Can you work these out from the model? Positions are in its coordinate system, mm. A direction names the side the tool comes from. Round coordinates to 2 decimals unless told otherwise and drop trailing zeros. Loops run counter-clockwise (first coordinate to the right, second up) from the corner with the lowest first, then second, coordinate; pieces in that order, holes last. Notation, with made-up numbers: (53.5, 8.5) -> (78.5, 8.5) arc R21 cw to (78.5, 34.5) -> close; hole circle Ø2 at (10.5, -16.5). An arc over 180 degrees is marked (long way). Write item = value, one per line.
from build123d import *

# Parameters (mm, degrees)
CYLINDER1707_R     = 1.5
CYLINDER1707_DEPTH = 60
CYLINDER1708_R     = 1.5
CYLINDER1708_DEPTH = 60
CYLINDER1704_R     = 1.5
CYLINDER1704_DEPTH = 60
CYLINDER1705_R     = 1.5
CYLINDER1705_DEPTH = 60
BOX662_W           = 6
BOX662_H           = 6
BOX662_DEPTH       = 2
BOX664_W           = 6
BOX664_H           = 6
BOX664_DEPTH       = 2
BOX663_W           = 6
BOX663_H           = 6
BOX663_DEPTH       = 2
BOX661_W           = 6
BOX661_H           = 6
BOX661_DEPTH       = 2
CYLINDER1700_R     = 5
CYLINDER1700_DEPTH = 5
CYLINDER1699_R     = 3
CYLINDER1699_DEPTH = 48
BOX660_W           = 42
BOX660_H           = 20
BOX660_DEPTH       = 6


with BuildPart() as obj1:
    # Cylinder1707 → Cylinder1707 (new body)
    with BuildSketch(Plane(origin=(18, 85, -57), x_dir=(1, 0, 0), z_dir=(0, 0, 1))):
        Circle(CYLINDER1707_R)
    extrude(amount=CYLINDER1707_DEPTH)


with BuildPart() as obj2:
    # Cylinder1708 → Cylinder1708 (new body)
    with BuildSketch(Plane(origin=(-18, 85, -57), x_dir=(1, 0, 0), z_dir=(0, 0, 1))):
        Circle(CYLINDER1708_R)
    extrude(amount=CYLINDER1708_DEPTH)


with BuildPart() as obj3:
    # Cylinder1704 → Cylinder1704 (new body)
    with BuildSketch(Plane(origin=(-18, 95, -57), x_dir=(1, 0, 0), z_dir=(0, 0, 1))):
        Circle(CYLINDER1704_R)
    extrude(amount=CYLINDER1704_DEPTH)


with BuildPart() as compound849:
    # Cylinder1705 → Cylinder1705 (new body)
    with BuildSketch(Plane(origin=(18, 95, -57), x_dir=(1, 0, 0), z_dir=(0, 0, 1))):
        Circle(CYLINDER1705_R)
    extrude(amount=CYLINDER1705_DEPTH)

    # Compound849: union obj1, obj2, obj3
    add(obj1.part)
    add(obj2.part)
    add(obj3.part)


with BuildPart() as krychle662:
    # Box662 → Box662 (new body)
    with BuildSketch(Plane(origin=(-21, 92, -56), x_dir=(1, 0, 0), z_dir=(0, 0, 1))):
        with Locations((3, 3)):
            Rectangle(BOX662_W, BOX662_H)
    extrude(amount=BOX662_DEPTH)


with BuildPart() as krychle664:
    # Box664 → Box664 (new body)
    with BuildSketch(Plane(origin=(15, 82, -56), x_dir=(1, 0, 0), z_dir=(0, 0, 1))):
        with Locations((3, 3)):
            Rectangle(BOX664_W, BOX664_H)
    extrude(amount=BOX664_DEPTH)


with BuildPart() as krychle663:
    # Box663 → Box663 (new body)
    with BuildSketch(Plane(origin=(15, 92, -56), x_dir=(1, 0, 0), z_dir=(0, 0, 1))):
        with Locations((3, 3)):
            Rectangle(BOX663_W, BOX663_H)
    extrude(amount=BOX663_DEPTH)


with BuildPart() as compound848:
    # Box661 → Box661 (new body)
    with BuildSketch(Plane(origin=(-21, 82, -56), x_dir=(1, 0, 0), z_dir=(0, 0, 1))):
        with Locations((3, 3)):
            Rectangle(BOX661_W, BOX661_H)
    extrude(amount=BOX661_DEPTH)

    # Compound848: union Krychle662, Krychle664, Krychle663
    add(krychle662.part)
    add(krychle664.part)
    add(krychle663.part)


with BuildPart() as compound848_1:
    # Compound848 placement: moved
    add(compound848.part.moved(Location((0, 0, 21))))


with BuildPart() as obj4:
    # Cylinder1700 → Cylinder1700 (new body)
    with BuildSketch(Plane(origin=(0, 90, -38), x_dir=(1, 0, 0), z_dir=(0, 0, 1))):
        Circle(CYLINDER1700_R)
    extrude(amount=CYLINDER1700_DEPTH)


with BuildPart() as obj5:
    # Cylinder1699 → Cylinder1699 (new body)
    with BuildSketch(Plane(origin=(0, 90, -55), x_dir=(1, 0, 0), z_dir=(0, 0, 1))):
        Circle(CYLINDER1699_R)
    extrude(amount=CYLINDER1699_DEPTH)


with BuildPart() as cut355:
    # Box660 → Box660 (new body)
    with BuildSketch(Plane(origin=(-21, 80, -38), x_dir=(1, 0, 0), z_dir=(0, 0, 1))):
        with Locations((21, 10)):
            Rectangle(BOX660_W, BOX660_H)
    extrude(amount=BOX660_DEPTH)

    # Cut347: cut obj5
    add(obj5.part, mode=Mode.SUBTRACT)

    # Cut346: cut obj4
    add(obj4.part, mode=Mode.SUBTRACT)

    # Cut349: cut Compound848
    add(compound848_1.part, mode=Mode.SUBTRACT)

    # Cut355: cut Compound849
    add(compound849.part, mode=Mode.SUBTRACT)


solid = cut355.part
1. I'm going to push a flat-ended pin straight in: pin 1 (2.5 mm diameter, centred on x = -18, y = 85, fed in from -Z). Where does the tip first touch, or does it pass through?
Entries:
pin_1 = through
2. Suppose I cut it at C-C, the plane z = -34.3. List the corners of the cut face in (x, y) for me.
Entries:
outline = (-21, 80) -> (21, 80) -> (21, 82) -> (15, 82) -> (15, 88) -> (21, 88) -> (21, 92) -> (15, 92) -> (15, 98) -> (21, 98) -> (21, 100) -> (-21, 100) -> (-21, 98) -> (-15, 98) -> (-15, 92) -> (-21, 92) -> (-21, 88) -> (-15, 88) -> (-15, 82) -> (-21, 82) -> close; hole circle Ø10 at (0, 90)
3. We'd pull the mould along Y, two halves only. Please class faces 1 (the flat face through (21, 90, -36)), 2 (the flat face through (-19.4, 86.4, -33)), 3 (the cylindrical face through (17.805, 86.487, -32.507)), 4 (the flat face through (0, 80, -35)): released by +Y, released by -Y, zero draft, split by the parting line, or undercut.
Entries:
face_1 = zero draft
face_2 = undercut
face_3 = undercut
face_4 = released by -Y
4. Suppose I cut it at B-B, the plane x = 18. List the corners of the cut face in (y, z) for me.
Entries:
outline = (80, -38) -> (83.5, -38) -> (83.5, -35) -> (82, -35) -> (82, -33) -> (83.5, -33) -> (83.5, -32) -> (80, -32) -> close; (86.5, -38) -> (93.5, -38) -> (93.5, -35) -> (92, -35) -> (92, -33) -> (93.5, -33) -> (93.5, -32) -> (86.5, -32) -> (86.5, -33) -> (88, -33) -> (88, -35) -> (86.5, -35) -> close; (96.5, -38) -> (100, -38) -> (100, -32) -> (96.5, -32) -> (96.5, -33) -> (98, -33) -> (98, -35) -> (96.5, -35) -> close
5. Suppose I cut it at A-A, the plane z = -36.35. List the corners of the cut face in (x, y) for me.
Entries:
outline = (-21, 80) -> (21, 80) -> (21, 100) -> (-21, 100) -> close; hole circle Ø3 at (-18, 85); hole circle Ø3 at (-18, 95); hole circle Ø10 at (0, 90); hole circle Ø3 at (18, 85); hole circle Ø3 at (18, 95)
6. I need wall thicknesses on line 1 (Y direction, x = 18, z = -32.7); line 2 (X direction, y = 95, z = -32.85); line 3 (X direction, y = 90, z = -32.6). Which ranges of each line are inside material? Lowest first, please. Write a range as [from, to].
Entries:
line_1 = [80, 83.5], [86.5, 93.5], [96.5, 100]
line_2 = [-21, -19.5], [-16.5, 16.5], [19.5, 21]
line_3 = [-21, -3], [3, 21]
7. For faces 5 (the cylindrical face through (-1.08, 85.12, -35.53)), 6 (the flat face through (-15, 95, -34)), 7 (the cylindrical face through (-18.195, 96.487, -32.507)), 8 (the flat face through (-5, 92, -38)), 9 (the flat face through (18, 88, -34)), which set-ups out of +Z, -Z, +X, -X, +Y, -Y let a thin tool reach every point of the face, with its end or its side?
Entries:
face_5 = -Z
face_6 = -X
face_7 = +Z, -Z
face_8 = -Z, +X, -X, +Y, -Y
face_9 = +X
8. Suppose I cut it at D-D, the plane y = 90. List the corners of the cut face in (x, z) for me.
Entries:
outline = (-21, -38) -> (-5, -38) -> (-5, -33) -> (-3, -33) -> (-3, -32) -> (-21, -32) -> close; (3, -33) -> (5, -33) -> (5, -38) -> (21, -38) -> (21, -32) -> (3, -32) -> close
